For this review, take the finished solid that the model builds, in its own axes (mm). Face numbers are marked on the shaded views. Round coordinates to 2 decimals unless told otherwise and drop trailing zeros. Loops run counter-clockwise (first coordinate to the right, second up) from the corner with the lowest first, then second, coordinate; pieces in that order, holes last. Notation, with made-up numbers: (65.25, 76) -> (118.25, 76) arc R34 cw to (118.25, 115) -> close; hole circle Ø8 at (20.25, 44). An arc over 180 degrees is marked (long way). One line per question, with ' | ' between items. Start each with the question number.
1. Consider section B-B (x = -5). Write out the cut boundary in (y, z), and give its area (3 significant figures).
2. Wall thickness on line 1 along Z through (x, y) = (-5.5, 2); line 2 along Z through (x, y) = (6, -0.75); line 3 along X through (y, z) = (2.75, -36.5): over which ranges is each line inside the solid? List them lowest first.
3. Draft analysis for pull direction Z (two halves, no side actions). For the marked faces 1 and 2, state which applies: pulls with the +Z half, pulls with the -Z half, needs draft (parallel to the pull), parting line crosses it, or undercut.
4. For pin 1 Ø1.5 at (x, z) = (14.5, -5.5) entering from +Y, flat-tipped, find the tip position at first contact; note if it passes through.
5. Consider section A-A (y = 1.25). Write out the cut boundary in (x, z).
6. Consider section D-D (x = 12). Write out the cut boundary in (y, z), and give its area (3 significant figures).
7. Consider section C-C (z = 44). Write out the cut boundary in (x, y).
```python
from build123d import *

# Parameters (mm, degrees)
F0_W     = 58.6
F0_H     = 123.8
F0_W_2   = 23.2377052307
F0_H_2   = 11.1885257065
F1_DEPTH = 3.55
F2_T     = -2.54
F3_R     = 5.08


with BuildPart() as f1:
    # F0 (on Front) → F1 (new body, symmetric)
    with BuildSketch(Plane.XZ):
        Rectangle(F0_W, F0_H)
        with Locations((-11.6188526154, 47.3360661417)):
            Rectangle(F0_W_2, F0_H_2, mode=Mode.SUBTRACT)
    extrude(amount=F1_DEPTH, both=True)

    # F2
    f2_openings = [f1.faces().sort_by_distance(p)[0] for p in [
        (0.431878, 3.55, -1.759504),
    ]]
    offset(amount=F2_T, openings=f2_openings, kind=Kind.INTERSECTION)

    # F3
    f3_edges = [f1.edges().sort_by_distance(p)[0] for p in [
        (29.3, 0, 61.9),
        (-29.3, 0, 61.9),
        (29.3, 0, -61.9),
        (-29.3, 0, -61.9),
    ]]
    fillet(f3_edges, radius=F3_R)


solid = f1.part
```
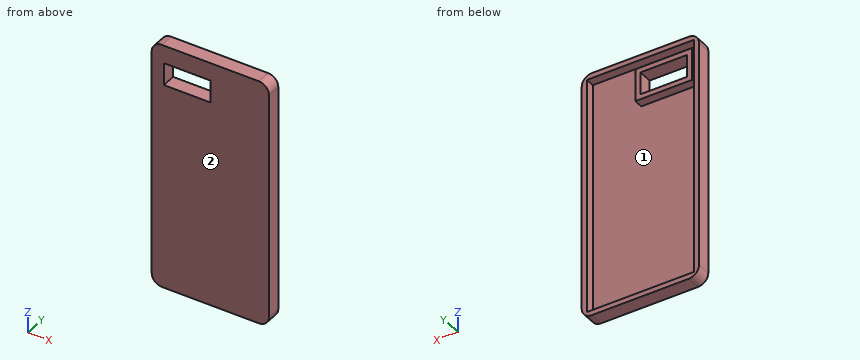
Answer block:
1) outline: (-3.55, -61.9) -> (3.55, -61.9) -> (3.55, -59.36) -> (-1.01, -59.36) -> (-1.01, 39.2) -> (3.55, 39.2) -> (3.55, 41.74) -> (-3.55, 41.74) -> close; (-3.55, 52.93) -> (3.55, 52.93) -> (3.55, 55.47) -> (-1.01, 55.47) -> (-1.01, 59.36) -> (3.55, 59.36) -> (3.55, 61.9) -> (-3.55, 61.9) -> close | area: 332 mm2
2) line 1: z = -61.9 to -59.36, 39.2 to 41.74, 52.93 to 55.47, 59.36 to 61.9 | line 2: z = -61.9 to -59.36, 59.36 to 61.9 | line 3: x = -29.3 to -26.76, 26.76 to 29.3
3) face 1: undercut | face 2: needs draft
4) pin 1: stops at y = -1.01
5) outline: (-29.3, -56.82) arc R5.08 ccw to (-24.22, -61.9) -> (24.22, -61.9) arc R5.08 ccw to (29.3, -56.82) -> (29.3, 56.82) arc R5.08 ccw to (24.22, 61.9) -> (-24.22, 61.9) arc R5.08 ccw to (-29.3, 56.82) -> close; (-25.78, 39.2) -> (2.54, 39.2) -> (2.54, 55.47) -> (-25.78, 55.47) -> close; hole (-26.76, -59.36) -> (26.76, -59.36) -> (26.76, 59.36) -> (-26.76, 59.36) -> close; hole (-23.24, 41.74) -> (0, 41.74) -> (0, 52.93) -> (-23.24, 52.93) -> close
6) outline: (-3.55, -61.9) -> (3.55, -61.9) -> (3.55, -59.36) -> (-1.01, -59.36) -> (-1.01, 59.36) -> (3.55, 59.36) -> (3.55, 61.9) -> (-3.55, 61.9) -> close | area: 338 mm2
7) outline: (-29.3, -3.55) -> (-23.24, -3.55) -> (-23.24, 3.55) -> (-25.78, 3.55) -> (-25.78, -1.01) -> (-26.76, -1.01) -> (-26.76, 3.55) -> (-29.3, 3.55) -> close; (0, -3.55) -> (29.3, -3.55) -> (29.3, 3.55) -> (26.76, 3.55) -> (26.76, -1.01) -> (2.54, -1.01) -> (2.54, 3.55) -> (0, 3.55) -> close
